```python
from build123d import *

# Parameters (mm, degrees)
SKETCH1_W           = 254
SKETCH1_H           = 127
BOSS_EXTRUDE1_DEPTH = 152.4
FILLET1_R           = 25.4
SKETCH3_R           = 3.81
CUT_EXTRUDE1_DEPTH  = 8.89


with BuildPart() as part:
    # Sketch1 → Boss-Extrude1 (new body)
    with BuildSketch(Plane(origin=(0, 0, 0), x_dir=(1, 0, 0), z_dir=(0, 1, 0))):
        Rectangle(SKETCH1_W, SKETCH1_H)
    extrude(amount=BOSS_EXTRUDE1_DEPTH)

    # Fillet1
    fillet1_edges = [part.edges().sort_by_distance(p)[0] for p in [
        (-127, 152.4, 0),
        (0, 152.4, 63.5),
        (127, 152.4, 0),
        (0, 0, 63.5),
        (-127, 0, 0),
        (0, 0, -63.5),
        (127, 0, 0),
        (127, 76.2, 63.5),
        (-127, 76.2, 63.5),
        (-127, 76.2, -63.5),
        (127, 76.2, -63.5),
        (0, 152.4, -63.5),
    ]]
    fillet(fillet1_edges, radius=FILLET1_R)

    # Sketch3 → Cut-Extrude1 (cut)
    with BuildSketch(Plane.XZ):
        with Locations((-50.8, 0)):
            Circle(SKETCH3_R)
    cut_extrude1 = extrude(amount=-CUT_EXTRUDE1_DEPTH, mode=Mode.SUBTRACT)

    # Mirror1: Cut-Extrude1 across plane
    add(cut_extrude1.mirror(Plane(origin=(0, 0, 0), x_dir=(0, 0, 1), z_dir=(1, 0, 0))), mode=Mode.SUBTRACT)


solid = part.part
```
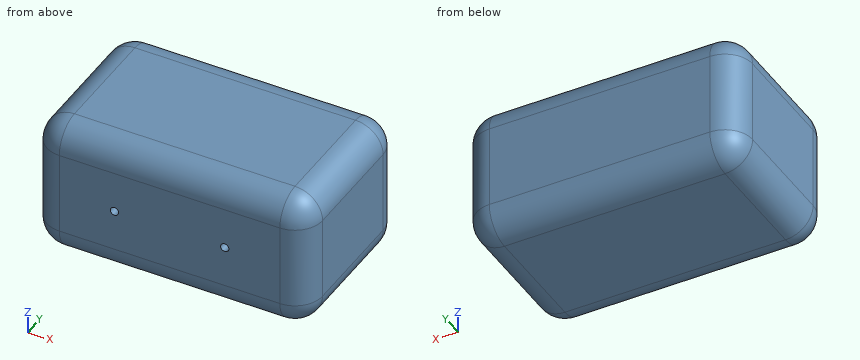
Geometry: final body of the model. Coordinates: model frame, mm. Round coordinates to 2 decimals unless told otherwise and drop trailing zeros. Write each loop counter-clockwise with the first axis right and the second up, starting at its lowest first coordinate (ties: lowest second). Pieces come first, ordered by that corner, then holes.
Item 1: Section query B-B (z = 0). Return loops of the section in (x, y), plus the area to 3 significant figures.
Item 2: Section query A-A (x = -50.8). Return loops of the section in (y, z), plus the area to 3 significant figures.
Item 3: Material intervals for L1, parallel to Z at x = -50.8, y = 2.5; L2, parallel to Z at x = 50.8, y = 4.25; L3, parallel to Y at x = 102.5, z = -56, sorted ascending.
Item 4: Section query C-C (y = 37). Return loops of the section in (x, z).
Item 5: Pin query (flat end, axial travel): P1, Ø4, axis at x = 52, z = 0, coming from the -Y side; P2, Ø8, axis at x = 52, z = -45, coming from the +Y side. Return the tip coordinate at first contact, or that it passes through.
Completed:
1. outline: (-127, 25.4) arc R25.4 ccw to (-101.6, 0) - (-54.61, 0) - (-54.61, 8.89) - (-46.99, 8.89) - (-46.99, 0) - (46.99, 0) - (46.99, 8.89) - (54.61, 8.89) - (54.61, 0) - (101.6, 0) arc R25.4 ccw to (127, 25.4) - (127, 127) arc R25.4 ccw to (101.6, 152.4) - (-101.6, 152.4) arc R25.4 ccw to (-127, 127) - close
1. area: 38,000 mm2
2. outline: (0, -38.1) arc R25.4 ccw to (25.4, -63.5) - (127, -63.5) arc R25.4 ccw to (152.4, -38.1) - (152.4, 38.1) arc R25.4 ccw to (127, 63.5) - (25.4, 63.5) arc R25.4 ccw to (0, 38.1) - (0, 3.81) - (8.89, 3.81) - (8.89, -3.81) - (0, -3.81) - close
2. area: 18,700 mm2
3. L1: z = -49.09 to -3.81, 3.81 to 49.09
3. L2: z = -52.17 to -3.81, 3.81 to 52.17
3. L3: y = 7.4 to 145
4. outline: (-127, -38.1) arc R25.4 ccw to (-101.6, -63.5) - (101.6, -63.5) arc R25.4 ccw to (127, -38.1) - (127, 38.1) arc R25.4 ccw to (101.6, 63.5) - (-101.6, 63.5) arc R25.4 ccw to (-127, 38.1) - close
5. P1: stops at y = 8.89
5. P2: stops at y = 152.23
